The listing builds one solid part. Answer for the finished solid, in the listing's coordinates (mm). A direction names the side the tool comes from. Round coordinates to 2 decimals unless told otherwise and drop trailing zeros. Loops run counter-clockwise (first coordinate to the right, second up) from the corner with the lowest first, then second, coordinate; pieces in that order, holes last. Notation, with made-up numbers: M -3,70 L 18,70 A21 cw 18,90 Z; hole C 85,14 d8. An arc over 180 degrees is marked long. Put each result on its own line as item: value. Start each with the question number.
(1) Section C-C, the plane z = -21 is taken. Determine the outline of the cut face in (x, y).
(2) Section B-B, the plane x = -38.5 is taken. Determine the outline of the cut face in (y, z).
(3) Section D-D, the plane x = 46.5 is taken. Determine the outline of the cut face in (y, z), then the cut area to 3 significant figures.
(4) Straight lines are drawn through the part: line 1 (X direction, y = -1.5, z = -8); line 2 (Z direction, x = 6.5, y = -1.4); line 3 (X direction, y = -1.3, z = -37). For each, find the intervals that lie inside material, in ascending order.
(5) Which of the six approach directions +Z, -Z, +X, -X, +Y, -Y give full straight-line access (tool end or side, diameter ignored) to faces 1 (the face through (4, -1, 0)), 2 (the face through (28, -1, -4.704))?
(6) Section A-A, the plane y = -1.7 is taken. Determine the outline of the cut face in (x, z).
(7) Determine the mould class of faces 3 (the face through (-48.846, -1, -28)), 4 (the face through (55.206, -1, -28)), 5 (the face through (-22, -1, -52.28)) for opening direction X: released by +X, released by -X, zero draft, split by the parting line, or undercut.
(8) Flat-ended cylindrical pins translate along their axes: P1, Ø1, axis at x = 12, y = -1.5, coming from the -Z side; P2, Ø0.8, axis at x = -17.5, y = -0.5, coming from the -Z side. Find the tip coordinate at first contact, or state that the pin passes through.
```python
from build123d import *

# Parameters (mm, degrees)
F1_DEPTH = 2.54


# Not quite as in the source:
# - a feature names something its author has since deleted; it is built from what else it names


with BuildPart() as f1:
    # F0 (on Front) → F1 (new body)
    with BuildSketch(Plane.XZ):
        Polygon((-45.7926876843, 0), (-48.8455332816, 0), (-48.8455332816, -56.6048510373), (-45.7926876843, -56.5824585276), (-45.7926876843, -52.2799864411), (-45.7926876843, -32.4403391187), (-45.7926876843, -28.3024255186), (-45.7926876843, -4.7043516129), align=None)
        Polygon((0, 0), (-45.7926876843, 0), (-45.7926876843, -4.7043516129), (0.0345062453, -4.7043516129), align=None)
        Polygon((-45.7926876843, -52.2799864411), (-45.7926876843, -56.5824585276), (5.5995524852, -56.2054983442), (5.5707590003, -52.2799864411), (0.3834717695, -52.2799864411), align=None)
        Polygon((5.1872872309, 0), (0, 0), (0.0345062453, -4.7043516129), (5.2217934762, -4.7043516129), align=None)
        Polygon((5.5707590003, -52.2799864411), (5.5995524852, -56.2054983442), (51.3895750046, -55.8696302204), (51.3895750046, -52.2799864411), align=None)
        Polygon((51.3895750046, 0), (5.1872872309, 0), (5.2217934762, -4.7043516129), (51.3895750046, -4.7043516129), align=None)
        Polygon((51.3895750046, -52.2799864411), (51.3895750046, -55.8696302204), (55.2056245506, -55.8416396379), (55.2056245506, 0), (51.3895750046, 0), (51.3895750046, -4.7043516129), (51.3895750046, -28.3024255186), align=None)
        Polygon((5.2217934762, -4.7043516129), (0.0345062453, -4.7043516129), (0.2379486892, -32.4403391187), (0.3834717695, -52.2799864411), (5.5707590003, -52.2799864411), align=None)
    extrude(amount=F1_DEPTH)


solid = f1.part
```
Recorded:
1. outline: M -48.85,-2.54 L -45.79,-2.54 L -45.79,0 L -48.85,0 Z; M 0.15,-2.54 L 5.34,-2.54 L 5.34,0 L 0.15,0 Z; M 51.39,-2.54 L 55.21,-2.54 L 55.21,0 L 51.39,0 Z
2. outline: M -2.54,-56.53 L 0,-56.53 L 0,-52.28 L -2.54,-52.28 Z; M -2.54,-4.7 L 0,-4.7 L 0,0 L -2.54,0 Z
3. outline: M -2.54,-55.91 L 0,-55.91 L 0,-52.28 L -2.54,-52.28 Z; M -2.54,-4.7 L 0,-4.7 L 0,0 L -2.54,0 Z
3. area: 21.2 mm²
4. line 1: x = -48.85 to -45.79, 0.06 to 5.25, 51.39 to 55.21
4. line 2: z = -56.2 to -52.28, -4.7 to 0
4. line 3: x = -48.85 to -45.79, 0.27 to 5.46, 51.39 to 55.21
5. face 1: +Z, +X, -X, +Y, -Y
5. face 2: +Y, -Y
6. outline: M -48.85,-56.6 L 55.21,-55.84 L 55.21,0 L -48.85,0 Z; hole M -45.79,-52.28 L 0.38,-52.28 L 0.03,-4.7 L -45.79,-4.7 Z; hole M 5.22,-4.7 L 5.57,-52.28 L 51.39,-52.28 L 51.39,-4.7 Z
7. face 3: released by -X
7. face 4: released by +X
7. face 5: undercut
8. P1: stops at z = -56.16
8. P2: stops at z = -56.38
